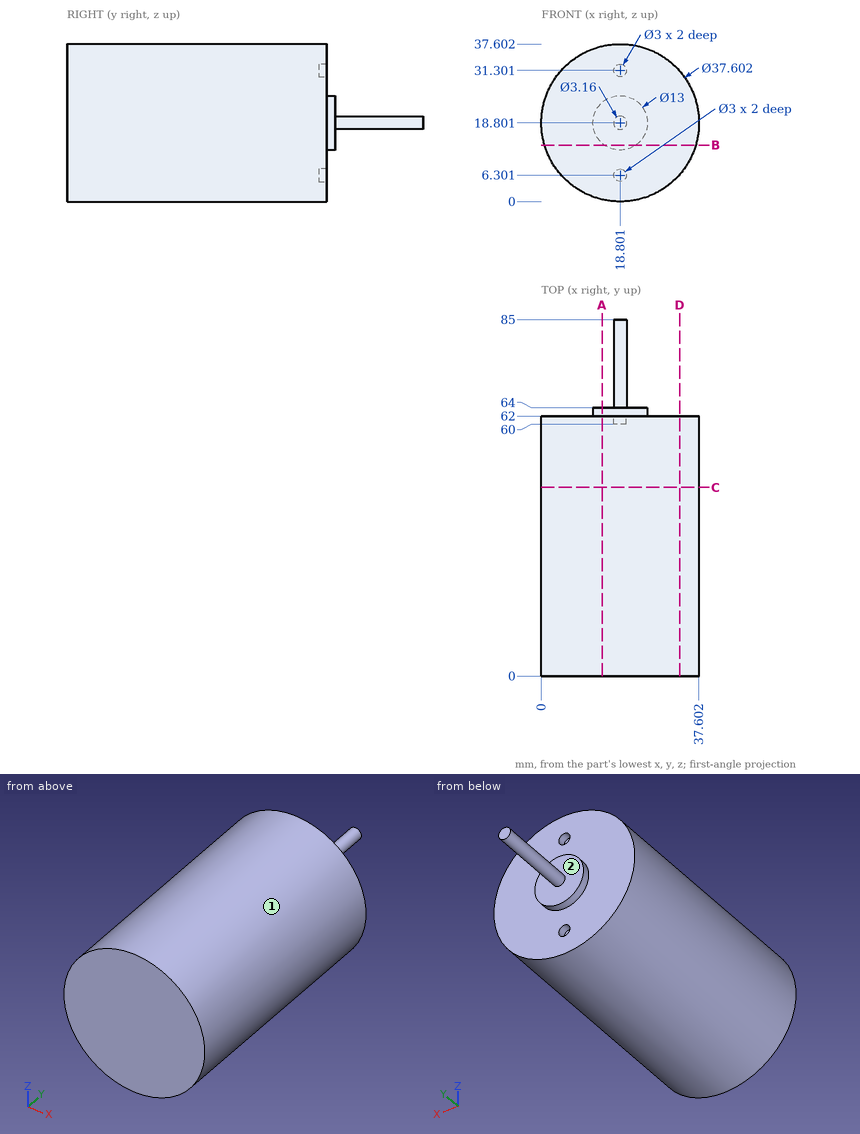
Verification items for this drawing (mm, ordinates from the low corner). A direction names the side the tool comes from. Round coordinates to 2 decimals unless told otherwise and drop trailing zeros. Loops run counter-clockwise (first coordinate to the right, second up) from the corner with the lowest first, then second, coordinate; pieces in that order, holes last. Notation, with made-up numbers: (49, 66) - (80, 66) arc R21 ccw to (80, 74) - close; hole circle Ø2 at (8, 42). An arc over 180 degrees is marked (long way). Write item = value, one per line.
Q1. Depth check by flat-ended pin: pin 1 (6 mm diameter, centred on x = 29, y = 59, fed in from +Z); pin 2 (8 mm diameter, centred on y = 39.5, z = 33, fed in from +X) (1 decimal); pin 3 (1.8 mm diameter, centred on x = 18.8, z = 31.3, fed in from +Y). Enter the tip coordinate at first touch or a pass-through.
Here are the results:
pin_1 = 36.17
pin_2 = 34.6
pin_3 = 60
Q2. Sectioned sample at D-D on x = 33. Record the boundary of the cut face in (y, z) (1 decimal).
Here are the results:
outline = (0, 6.5) - (62, 6.5) - (62, 31.1) - (0, 31.1) - close
Q3. Sectioned sample at B-B on z = 13.5. Record the boundary of the cut face in (x, y).
Here are the results:
outline = (0.76, 0) - (36.84, 0) - (36.84, 62) - (22.56, 62) - (22.56, 64) - (15.04, 64) - (15.04, 62) - (0.76, 62) - close
Q4. Sectioned sample at A-A on x = 14.5. Record the boundary of the cut face in (y, z).
Here are the results:
outline = (0, 0.5) - (62, 0.5) - (62, 13.93) - (64, 13.93) - (64, 23.67) - (62, 23.67) - (62, 37.1) - (0, 37.1) - close
Q5. Tool access check on the marked faces 1 and 2. Record the directions out of +Z, -Z, +X, -X, +Y, -Y that give a thin tool (end or side, any length) a straight path to the whole face; none if there is none.
Here are the results:
face_1 = +Y, -Y
face_2 = +Y
Q6. Material ranges on L1, parallel to Y at x = 2.5, z = 18; L2, parallel to X at y = 39.5, z = 19; L3, parallel to Y at x = 14, z = 19.5, recorded low to high.
Here are the results:
L1 = 0 to 62
L2 = 0 to 37.6
L3 = 0 to 64
Q7. Sectioned sample at C-C on y = 45. Record the boundary of the cut face in (x, z).
Here are the results:
outline = circle Ø37.6 at (18.8, 18.8)
